```python
from build123d import *

# Parameters (mm, degrees)
CROQUIS2_W               = 30
CROQUIS2_H               = 31
CROQUIS2_W_2             = 3.1
CROQUIS2_H_2             = 7
CROQUIS2_W_3             = 2.5
CROQUIS2_R               = 2
SALIENTE_EXTRUIR1_DEPTH  = 3
CORTAR_EXTRUIR1_START    = 2
CROQUIS2_4_R             = 2.5
CROQUIS2_4_R_2           = 2
CORTAR_EXTRUIR1_DEPTH    = 1
CROQUIS2_5_W             = 14.15
CROQUIS2_5_H             = 10.7
SALIENTE_EXTRUIR2_DEPTH  = 2
CROQUIS2_7_W             = 7.9
CROQUIS2_7_H             = 2
SALIENTE_EXTRUIR3_DEPTH  = 119.5
CROQUIS2_9_W             = 4.8
CROQUIS2_9_H             = 7
CROQUIS2_9_W_2           = 6.3
SALIENTE_EXTRUIR4_DEPTH  = 0.6
SALIENTE_EXTRUIR5_DEPTH  = 8.2
CROQUIS3_R               = 0.95
SALIENTE_EXTRUIR6_DEPTH  = 0.4
REDONDEO1_R              = 0.25
REDONDEO1_OF_SIMETR_A1_R = 0.25
REDONDEO2_R              = 2.5


with BuildPart() as part:
    # Croquis2 → Saliente-Extruir1 (new body)
    with BuildSketch(Plane(origin=(0, 0, 0), x_dir=(0, 1, 0), z_dir=(0, 0, 1))):
        Rectangle(CROQUIS2_W, CROQUIS2_H)
        with Locations((9.95, -6.5)):
            Rectangle(CROQUIS2_W_2, CROQUIS2_H_2, mode=Mode.SUBTRACT)
        with Locations((0.85, -6.5)):
            Rectangle(CROQUIS2_W_3, CROQUIS2_H_2, mode=Mode.SUBTRACT)
        with Locations((-6.75, -6.5)):
            Rectangle(CROQUIS2_W_2, CROQUIS2_H_2, mode=Mode.SUBTRACT)
        with Locations(Location((9.15, 9, 0), (0, 0, 270))):
            Circle(CROQUIS2_R, mode=Mode.SUBTRACT)
    extrude(amount=SALIENTE_EXTRUIR1_DEPTH)

    # Croquis2<4> → Cortar-Extruir1 (cut)
    with BuildSketch(Plane(origin=(0, 0, 0), x_dir=(0, 1, 0), z_dir=(0, 0, 1)).offset(CORTAR_EXTRUIR1_START)):
        with Locations(Location((9.15, 9, 0), (0, 0, 270))):
            Circle(CROQUIS2_4_R)
        with Locations(Location((9.15, 9, 0), (0, 0, 270))):
            Circle(CROQUIS2_4_R_2, mode=Mode.SUBTRACT)
    extrude(amount=CORTAR_EXTRUIR1_DEPTH, mode=Mode.SUBTRACT)

    # Croquis2<5> → Saliente-Extruir2 (add)
    with BuildSketch(Plane(origin=(0, 0, 0), x_dir=(0, 1, 0), z_dir=(0, 0, 1))):
        with Locations((-3.775, 7.85)):
            Rectangle(CROQUIS2_5_W, CROQUIS2_5_H)
    extrude(amount=-SALIENTE_EXTRUIR2_DEPTH)

    # Croquis2<7> → Saliente-Extruir3 (add)
    with BuildSketch(Plane(origin=(0, 0, 0), x_dir=(0, 1, 0), z_dir=(0, 0, 1))):
        with Locations((0, -14.5)):
            Rectangle(CROQUIS2_7_W, CROQUIS2_7_H)
    extrude(amount=-SALIENTE_EXTRUIR3_DEPTH)

    # Croquis2<9> → Saliente-Extruir4 (add)
    with BuildSketch(Plane(origin=(0, 0, 0), x_dir=(0, 1, 0), z_dir=(0, 0, 1))):
        with Locations((-2.8, -6.5)):
            Rectangle(CROQUIS2_9_W, CROQUIS2_9_H)
        with Locations((5.25, -6.5)):
            Rectangle(CROQUIS2_9_W_2, CROQUIS2_9_H)
    extrude(amount=-SALIENTE_EXTRUIR4_DEPTH)

    # Croquis2<11> → Saliente-Extruir5 (add)
    with BuildSketch(Plane(origin=(0, 0, 0), x_dir=(0, 1, 0), z_dir=(0, 0, 1))):
        Polygon((-8.3, -3), (-8.3, -1), (11.5, -1), (11.5, -3), (8.4, -3), (2.1, -3), (-0.4, -3), (-5.2, -3), align=None)
        Polygon((11.5, -10), (11.5, -12), (-8.3, -12), (-8.3, -10), (-5.2, -10), (-0.4, -10), (2.1, -10), (8.4, -10), align=None)
    extrude(amount=-SALIENTE_EXTRUIR5_DEPTH)

    # Croquis3 → Saliente-Extruir6 (add)
    with BuildSketch(Plane.YZ.offset(3)):
        with Locations(Location((-3.1, -3.505, 0), (0, 0, 180))):
            Circle(CROQUIS3_R)
        with BuildLine():
            Line((6.769966215, -2.63), (6.030033785, -2.63))
            ThreePointArc((6.030033785, -2.63), (5.45, -3.505), (6.030033785, -4.38))
            Line((6.030033785, -4.38), (6.769966215, -4.38))
            ThreePointArc((6.769966215, -4.38), (7.35, -3.505), (6.769966215, -2.63))
        make_face()
    saliente_extruir6 = extrude(amount=SALIENTE_EXTRUIR6_DEPTH)

    # Redondeo1
    redondeo1_edges = [part.edges().sort_by_distance(p)[0] for p in [
        (3.4, -2.15, -3.505),
        (3.4, 7.35, -3.505),
        (3.4, 6.4, -2.63),
        (3.4, 5.45, -3.505),
        (3.4, 6.4, -4.38),
    ]]
    fillet(redondeo1_edges, radius=REDONDEO1_R)

    # Simetría1: Saliente-Extruir6 across plane
    add(saliente_extruir6.mirror(Plane(origin=(6.5, 0, 0), x_dir=(0, 0, 1), z_dir=(1, 0, 0))))

    # Redondeo1 of Simetría1
    redondeo1_of_simetr_a1_edges = [part.edges().sort_by_distance(p)[0] for p in [
        (9.6, -2.15, -3.505),
        (9.6, 7.35, -3.505),
        (9.6, 6.4, -2.63),
        (9.6, 5.45, -3.505),
        (9.6, 6.4, -4.38),
    ]]
    fillet(redondeo1_of_simetr_a1_edges, radius=REDONDEO1_OF_SIMETR_A1_R)

    # Redondeo2
    redondeo2_edges = [part.edges().sort_by_distance(p)[0] for p in [
        (-15.5, -15, 1.5),
        (-15.5, 15, 1.5),
        (15.5, 15, 1.5),
        (15.5, -15, 1.5),
    ]]
    fillet(redondeo2_edges, radius=REDONDEO2_R)


solid = part.part
```
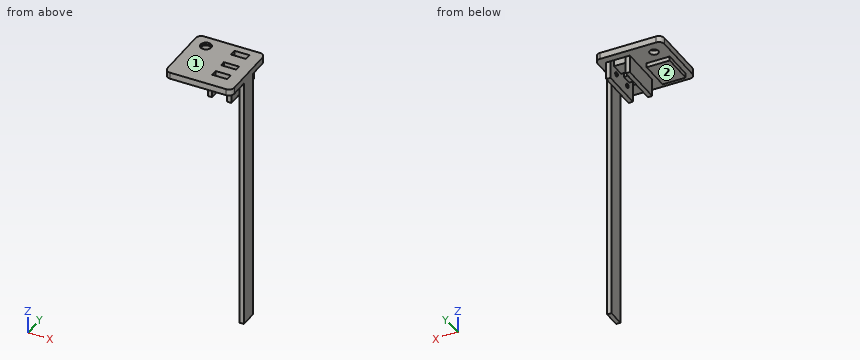
The listing builds one solid part. Answer for the finished solid, in the listing's coordinates (mm). Face numbers are marked on the shaded views. A direction names the side the tool comes from. Coordinates: 2 decimals unless noted, no trailing zeros. Write each loop counter-clockwise with the first axis right and the second up, starting at its lowest first coordinate (ties: lowest second). Pieces come first, ordered by that corner, then holes.
Q1. Which of the six approach directions +Z, -Z, +X, -X, +Y, -Y give full straight-line access (tool end or side, diameter ignored) to the marked faces 1 and 2?
Returned:
face 1: +Z, +X, -X, +Y, -Y
face 2: -Z, -X, +Y, -Y
Q2. Given P1, Ø1.5, axis at x = 7.5, y = 8.5, coming from the -Z side; P2, Ø5, axis at y = 5, z = -100.5, coming from the -X side; P3, Ø1, axis at x = 11.5, z = -4.5, coming from the +Y side; P4, Ø5, axis at y = -7, z = -37.5, coming from the +X side, each flat-ended and moving along its own axis, determine where each tip first touches the part or whether it passes through.
Returned:
P1: stops at z = -0.6
P2: stops at x = 13.5
P3: stops at y = 11.5
P4: passes through
Q3. Section A-A, the plane x = 7.5 is taken. Write down the section's boundary in (y, z).
Returned:
outline: (-15, 0) - (-8.3, 0) - (-8.3, 3) - (-15, 3) - close; (-5.2, -0.6) - (-0.4, -0.6) - (-0.4, 3) - (-5.2, 3) - close; (2.1, -0.6) - (8.4, -0.6) - (8.4, 3) - (2.1, 3) - close; (11.5, 0) - (15, 0) - (15, 3) - (11.5, 3) - close
Q4. Section D-D, the plane z = -23 is taken. Write down the section's boundary in (x, y).
Returned:
outline: (13.5, -3.95) - (15.5, -3.95) - (15.5, 3.95) - (13.5, 3.95) - close
Q5. Section C-C, the plane x = -4 is taken. Write down the section's boundary in (y, z).
Returned:
outline: (-15, 0) - (-10.85, 0) - (-10.85, -2) - (3.3, -2) - (3.3, 0) - (15, 0) - (15, 3) - (-15, 3) - close
Q6. Section B-B, the plane x = -9 is taken. Write down the section's boundary in (y, z), then the cut area to 3 significant figures.
Returned:
outline: (-15, 0) - (-10.85, 0) - (-10.85, -2) - (3.3, -2) - (3.3, 0) - (7.15, 0) - (7.15, 2) - (6.65, 2) - (6.65, 3) - (-15, 3) - close; (11.15, 0) - (15, 0) - (15, 3) - (11.65, 3) - (11.65, 2) - (11.15, 2) - close
area: 105 mm2
Q7. Find the intervals of material crossed by line 1 along Y through (x, z) = (-9, 2.2); line 2 along X through (y, z) = (-6.5, -7); line 3 along Y through (x, z) = (-9, 0.7), in increasing order.
Returned:
line 1: y = -15 to 6.65, 11.65 to 15
line 2: x = 1 to 3, 10 to 12
line 3: y = -15 to 7.15, 11.15 to 15
